Part model, mm, in its own coordinate system. Face numbers are marked on the shaded views. A direction names the side the tool comes from. Give positions to 0.01 mm unless a question says otherwise; leave off trailing zeros. Write each loop counter-clockwise with the first axis right and the second up, starting at its lowest first coordinate (ties: lowest second). Pieces come first, ordered by that corner, then holes.
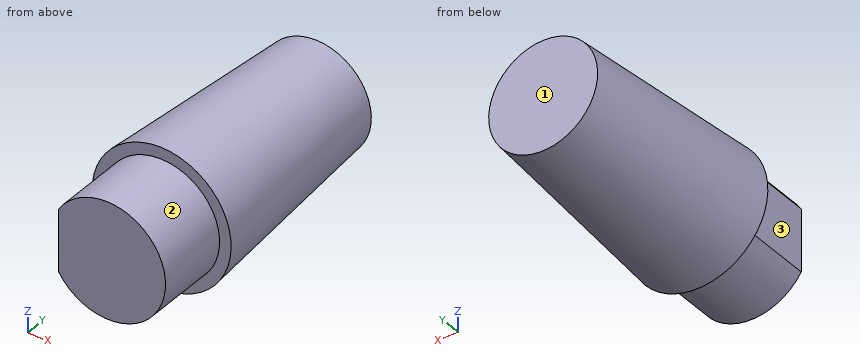
from build123d import *

# Parameters (mm, degrees)
SKETCH1_R           = 15.35
BOSS_EXTRUDE1_DEPTH = 63.9
SKETCH2_R           = 15.35
CUT_EXTRUDE1_DEPTH  = 16.5
DRAFT3_ANGLE        = -4


with BuildPart() as part:
    # Sketch1 → Boss-Extrude1 (new body)
    with BuildSketch(Plane(origin=(0, 0, 0), x_dir=(1, 0, 0), z_dir=(0, 1, 0))):
        with Locations(Location((0, 0, 0), (0, 0, 270))):
            Circle(SKETCH1_R)
    extrude(amount=BOSS_EXTRUDE1_DEPTH)

    # Sketch2 → Cut-Extrude1 (cut)
    with BuildSketch(Plane.XZ):
        with Locations(Location((0, 0, 0), (0, 0, 270))):
            Circle(SKETCH2_R)
        with BuildLine():
            Line((-10.8, -6.870225615), (-10.8, 6.870225615))
            ThreePointArc((-10.8, 6.870225615), (12.8, 0), (-10.8, -6.870225615))
        make_face(mode=Mode.SUBTRACT)
    extrude(amount=-CUT_EXTRUDE1_DEPTH, mode=Mode.SUBTRACT)

    # Draft3
    draft3_faces = [part.faces().sort_by_distance(p)[0] for p in [
        (0, 40.2, -15.35),
    ]]
    draft(draft3_faces, Plane(origin=(0, 16.5, 0), x_dir=(0, 0, -1), z_dir=(0, -1, 0)), DRAFT3_ANGLE)


solid = part.part
1) Saw through at C-C (y = 48.5). Write the cut outline in (x, z).
Check result:
outline: circle Ø26.22 at (0, 0)
2) Saw through at A-A (x = 0). Write the cut outline in (y, z).
Check result:
outline: (0, -12.8) - (16.5, -12.8) - (16.5, -15.35) - (63.9, -12.04) - (63.9, 12.04) - (16.5, 15.35) - (16.5, 12.8) - (0, 12.8) - close
3) Flat gauge pins, fed straight in: P1, Ø12, axis at y = 42.5, z = -10, coming from the -X side; P2, Ø11, axis at y = 10, z = 1.5, coming from the -X side; P3, Ø6, axis at x = -4, y = 55.5, coming from the -Z side. Where does each tip first touch, or does it go through?
Check result:
P1: stops at x = -12.98
P2: stops at x = -10.8
P3: stops at z = -12.65
4) Saw through at D-D (y = 55.5). Write the cut outline in (x, z).
Check result:
outline: circle Ø25.25 at (0, 0)
5) 3-axis set-ups, long thin cutter, end or side, ignore diameter. For the marked faces 1, 2 and 3: which of +Z, -Z, +X, -X, +Y, -Y reach the whole face in a straight line?
Check result:
face 1: +Z, -Z, +X, -X, +Y
face 2: -Y
face 3: +Z, -Z, -X, -Y
6) Saw through at B-B (z = 0). Write the cut outline in (x, y).
Check result:
outline: (-15.35, 16.5) - (-10.8, 16.5) - (-10.8, 0) - (12.8, 0) - (12.8, 16.5) - (15.35, 16.5) - (12.04, 63.9) - (-12.04, 63.9) - close
7) Drill centre lines: L1, parallel to X at y = 50.5, z = 2; L2, parallel to X at y = 31, z = 6; L3, parallel to Z at x = 4.5, y = 41. Where is each one in solid material? Low to high.
Check result:
L1: x = -12.82 to 12.82
L2: x = -13.02 to 13.02
L3: z = -12.87 to 12.87
